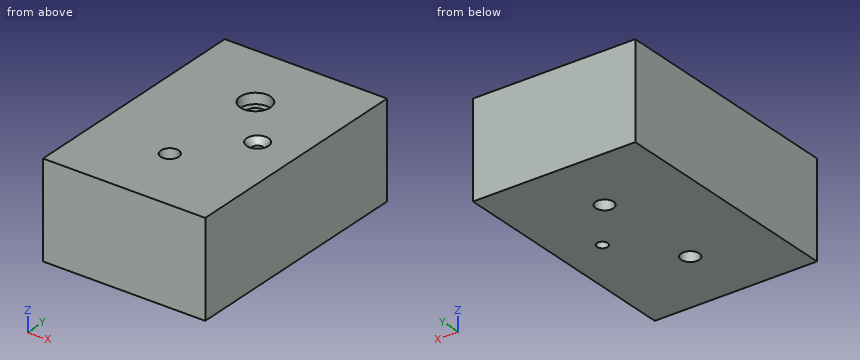
from build123d import *

# Parameters (mm, degrees)
SKETCH1_W                                     = 300
SKETCH1_H                                     = 450
BOSS_EXTRUDE1_DEPTH                           = 175
CBORE_FOR_M30_HEX_HEAD_CAP_SCREW1_D           = 33
CBORE_FOR_M30_HEX_HEAD_CAP_SCREW1_CBORE_D     = 56.12
CBORE_FOR_M30_HEX_HEAD_CAP_SCREW1_CBORE_DEPTH = 19.48
M36X3_0_TAPPED_HOLE1_D                        = 33
HOLE1_D                                       = 20
HOLE1_CSINK_D                                 = 40
HOLE1_CSINK_ANGLE                             = 82


with BuildPart() as part:
    # Sketch1 → Boss-Extrude1 (new body)
    with BuildSketch(Plane.XY):
        with Locations((150, 225)):
            Rectangle(SKETCH1_W, SKETCH1_H)
    extrude(amount=BOSS_EXTRUDE1_DEPTH)

    # CBORE for M30 Hex Head Cap Screw1 (through all)
    with Locations(Plane.XY.offset(175)):
        with Locations((150, 325)):
            CounterBoreHole(CBORE_FOR_M30_HEX_HEAD_CAP_SCREW1_D / 2, CBORE_FOR_M30_HEX_HEAD_CAP_SCREW1_CBORE_D / 2, CBORE_FOR_M30_HEX_HEAD_CAP_SCREW1_CBORE_DEPTH)

    # M36x3.0 Tapped Hole1 (through all)
    with Locations(Plane.XY.offset(175)):
        with Locations((141.698240344, 124.123333408)):
            Hole(M36X3_0_TAPPED_HOLE1_D / 2)

    # Hole1 (through all)
    with Locations(Plane.XY.offset(175)):
        with Locations((225, 230)):
            CounterSinkHole(HOLE1_D / 2, HOLE1_CSINK_D / 2, counter_sink_angle=HOLE1_CSINK_ANGLE)


solid = part.part
Work out the finished part from the listing and answer in its coordinate system (mm). Give positions to 0.01 mm unless a question says otherwise; leave off trailing zeros. Loops run counter-clockwise (first coordinate to the right, second up) from the corner with the lowest first, then second, coordinate; pieces in that order, holes last. Notation, with made-up numbers: (-19, 73) -> (-13, 73) arc R26 cw to (-13, 107) -> close; hole circle Ø1 at (16.25, -39.75). An arc over 180 degrees is marked (long way). Use a Markdown table: item, result. Add a question column.
1. Section A-A on y = 230 is taken. Determine the outline of the cut face in (x, z).
2. Section D-D on y = 325 is taken. Determine the outline of the cut face in (x, z).
3. Find the intervals of material crossed by probe 1 along Y at (x, z) = (150, 168.5); probe 2 along X at (y, z) = (230, 82); probe 3 along Y at (x, z) = (150, 68), in increasing order.
4. Flat-ended cylindrical pins translate along their axes: pin 1 Ø4 at (x, y) = (170.5, 262) entering from -Z; pin 2 Ø18 at (x, y) = (225, 230) entering from -Z; pin 3 Ø17 at (x, y) = (158.5, 334) entering from +Z. Find the tip coordinate at first contact, or state that the pin passes through.
5. Section B-B on x = 225 is taken. Determine the outline of the cut face in (y, z), and give its area (3 significant figures).
6. Section C-C on x = 150 is taken. Determine the outline of the cut face in (y, z), and give its area (3 significant figures).
Results below:
| question | item | result |
|---|---|---|
| 1 | outline | (0, 0) -> (215, 0) -> (215, 163.5) -> (205, 175) -> (0, 175) -> close; (235, 0) -> (300, 0) -> (300, 175) -> (245, 175) -> (235, 163.5) -> close |
| 2 | outline | (0, 0) -> (133.5, 0) -> (133.5, 155.52) -> (121.94, 155.52) -> (121.94, 175) -> (0, 175) -> close; (166.5, 0) -> (300, 0) -> (300, 175) -> (178.06, 175) -> (178.06, 155.52) -> (166.5, 155.52) -> close |
| 3 | probe 1 | y = 0 to 109.86, 138.38 to 296.94, 353.06 to 450 |
| 3 | probe 2 | x = 0 to 215, 235 to 300 |
| 3 | probe 3 | y = 0 to 109.86, 138.38 to 308.5, 341.5 to 450 |
| 4 | pin 1 | stops at z = 0 |
| 4 | pin 2 | passes through |
| 4 | pin 3 | stops at z = 155.52 |
| 5 | outline | (0, 0) -> (220, 0) -> (220, 163.5) -> (210, 175) -> (0, 175) -> close; (240, 0) -> (450, 0) -> (450, 175) -> (250, 175) -> (240, 163.5) -> close |
| 5 | area | 75,100 mm^2 |
| 6 | outline | (0, 0) -> (109.86, 0) -> (109.86, 175) -> (0, 175) -> close; (138.38, 0) -> (308.5, 0) -> (308.5, 155.52) -> (296.94, 155.52) -> (296.94, 175) -> (138.38, 175) -> close; (341.5, 0) -> (450, 0) -> (450, 175) -> (353.06, 175) -> (353.06, 155.52) -> (341.5, 155.52) -> close |
| 6 | area | 67,500 mm^2 |
